```python
from build123d import *

# Parameters (mm, degrees)
F0_R     = 20
F1_DEPTH = 5
F2_R     = 11
F3_DEPTH = 8
F4_R     = 9.9
F5_DEPTH = 12
F6_R     = 7.925
F7_DEPTH = 10
F9_D     = 11.92
F11_D    = 4.5


with BuildPart() as f1:
    # F0 (on Top) → F1 (new body)
    with BuildSketch(Plane.XY):
        Circle(F0_R)
    extrude(amount=F1_DEPTH)

    # F2 (on face) → F3 (join)
    with BuildSketch(Plane.XY.offset(5)):
        Circle(F2_R)
    extrude(amount=F3_DEPTH)

    # F4 (on face) → F5 (join)
    with BuildSketch(Plane.XY.offset(13)):
        Circle(F4_R)
    extrude(amount=F5_DEPTH)

    # F6 (on face) → F7 (join)
    with BuildSketch(Plane(origin=(0, 0, 0), x_dir=(1, 0, 0), z_dir=(0, 0, -1))):
        Circle(F6_R)
    extrude(amount=F7_DEPTH)

    # F9 (through all)
    with Locations(Plane.XY.offset(25)):
        with Locations((0, 0)):
            Hole(F9_D / 2)

    # F11 (through all)
    with Locations(Plane(origin=(0, 0, 0), x_dir=(1, 0, 0), z_dir=(0, 0, -1))):
        with Locations((0, -15), (0, 15)):
            Hole(F11_D / 2)


solid = f1.part
```
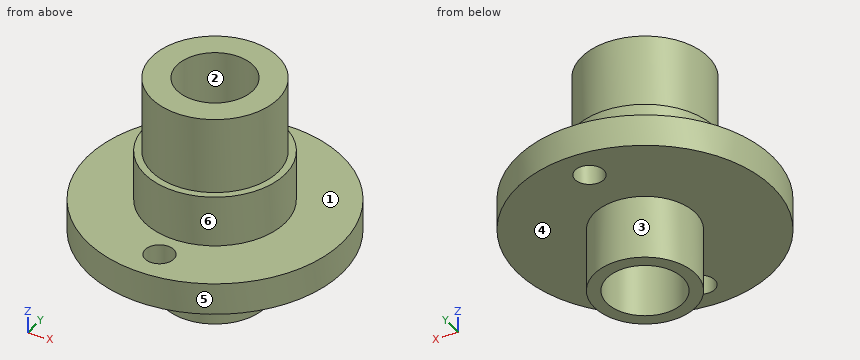
CAD build for the part. Positions are in the model's coordinates, mm. Face numbers are marked on the shaded views. A direction names the side the tool comes from. Round coordinates to 2 decimals unless told otherwise and drop trailing zeros. Loops run counter-clockwise (first coordinate to the right, second up) from the corner with the lowest first, then second, coordinate; pieces in that order, holes last. Notation, with made-up numbers: M 35,39 L 48,39 A7 ccw 48,45 Z; hole C 48.5,41.25 d8. An arc over 180 degrees is marked long. Return JSON: item names as keys, results as strings. Group by question number.
(1) Saw through at A-A, the plane y = 0. List the corners of the cut face in (x, z) (3 decimals), and give its area (3 significant figures).
(2) Saw through at D-D, the plane x = -5. List the corners of the cut face in (y, z).
(3) Tool access for the marked faces 4, 5 and 6: list every direction of +Z, -Z, +X, -X, +Y, -Y with a clear straight run to the whole face (end or side of a thin tool).
(4) Drop flat-ended pins along their axis: P1, Ø6, axis at x = 7.5, z = -2, coming from the +Y side; P2, Ø10, axis at x = 12, y = -14.5, coming from the -Z side; P3, Ø4, axis at y = 10.5, z = 4.5, coming from the +X side. Give the stop position or say it passes through.
(5) Saw through at C-C, the plane z = 6. List the corners of the cut face in (x, y), and give its area (3 significant figures).
(6) Wall check: probe 1 along Y at (x, z) = (0, 3); probe 2 along Y at (x, z) = (0, 11); probe 3 along Z at (x, y) = (-2.5, -15). Give the ranges that are in metal, low to high. Write a range as [from, to].
(7) Mould opens along Y. For the marked faces 1, 2 and 3 say: +Y half, -Y half, draft (parallel to the pull), parting line (faces both ways), or undercut.
(8) Saw through at B-B, the plane x = 0. List the corners of the cut face in (y, z) (3 decimals), and give its area (3 significant figures).
Answer list:
{
 "1": {"outline": "M -20,0 L -7.925,0 L -7.925,-10 L -5.96,-10 L -5.96,25 L -9.9,25 L -9.9,13 L -11,13 L -11,5 L -20,5 Z; M 5.96,-10 L 7.925,-10 L 7.925,0 L 20,0 L 20,5 L 11,5 L 11,13 L 9.9,13 L 9.9,25 L 5.96,25 Z", "area": "355 mm2"},
 "2": {"outline": "M -19.36,0 L -6.15,0 L -6.15,-10 L -3.24,-10 L -3.24,25 L -8.54,25 L -8.54,13 L -9.8,13 L -9.8,5 L -19.36,5 Z; M 3.24,-10 L 6.15,-10 L 6.15,0 L 19.36,0 L 19.36,5 L 9.8,5 L 9.8,13 L 8.54,13 L 8.54,25 L 3.24,25 Z"},
 "3": {"face 4": "-Z", "face 5": "+Z, -Z", "face 6": "+Z"},
 "4": {"P1": "y = 19.29", "P2": "z = 0", "P3": "x = 18.1"},
 "5": {"outline": "C 0,0 d22; hole C 0,0 d11.92", "area": "269 mm2"},
 "6": {"probe 1": "[-20, -17.25], [-12.75, -5.96], [5.96, 12.75], [17.25, 20]", "probe 2": "[-11, -5.96], [5.96, 11]", "probe 3": "[0, 5]"},
 "7": {"face 1": "draft", "face 2": "undercut", "face 3": "parting line"},
 "8": {"outline": "M -20,0 L -17.25,0 L -17.25,5 L -20,5 Z; M -12.75,0 L -7.925,0 L -7.925,-10 L -5.96,-10 L -5.96,25 L -9.9,25 L -9.9,13 L -11,13 L -11,5 L -12.75,5 Z; M 5.96,-10 L 7.925,-10 L 7.925,0 L 12.75,0 L 12.75,5 L 11,5 L 11,13 L 9.9,13 L 9.9,25 L 5.96,25 Z; M 17.25,0 L 20,0 L 20,5 L 17.25,5 Z", "area": "310 mm2"}
}
